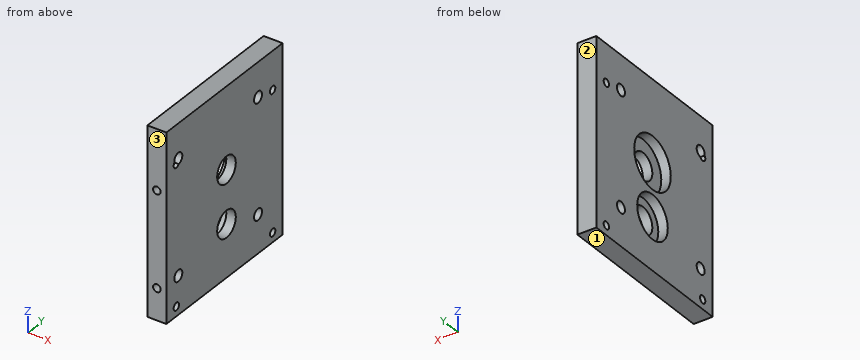
```python
from build123d import *

# Parameters (mm, degrees)
SKETCH1_W           = 20
SKETCH1_H           = 196
BOSS_EXTRUDE1_DEPTH = 175
SKETCH2_R           = 27.5
SKETCH2_R_2         = 23
CUT_EXTRUDE1_DEPTH  = 10
SKETCH3_R           = 14
CUT_EXTRUDE2_DEPTH  = 201.820815654
SKETCH4_R           = 4
CUT_EXTRUDE3_DEPTH  = 202.566366242
SKETCH5_R           = 6
CUT_EXTRUDE4_DEPTH  = 202.566366242
SKETCH6_R           = 4
CUT_EXTRUDE6_DEPTH  = 12


with BuildPart() as part:
    # Sketch1 → Boss-Extrude1 (new body)
    with BuildSketch(Plane(origin=(114, 0, 0), x_dir=(1, 0, 0), z_dir=(0, 1, 0))):
        with Locations((-114, 0)):
            Rectangle(SKETCH1_W, SKETCH1_H)
    extrude(amount=BOSS_EXTRUDE1_DEPTH)

    # Sketch2 → Cut-Extrude1 (cut)
    with BuildSketch(Plane.ZY.offset(10)):
        with Locations((12.5, 90.5)):
            Circle(SKETCH2_R)
        with Locations((-43, 90.5)):
            Circle(SKETCH2_R_2)
    extrude(amount=-CUT_EXTRUDE1_DEPTH, mode=Mode.SUBTRACT)

    # Sketch3 → Cut-Extrude2 (cut, through all)
    with BuildSketch(Plane.ZY):
        with Locations((12.5, 90.5)):
            Circle(SKETCH3_R)
        with Locations((-43, 90.5)):
            Circle(SKETCH3_R)
    extrude(amount=-CUT_EXTRUDE2_DEPTH, mode=Mode.SUBTRACT)

    # Sketch4 → Cut-Extrude3 (cut, through all)
    with BuildSketch(Plane.ZY.offset(10)):
        with Locations((58, 15)):
            Circle(SKETCH4_R)
        with Locations((-88, 15)):
            Circle(SKETCH4_R)
        with Locations((-88, 160)):
            Circle(SKETCH4_R)
        with Locations((58, 160)):
            Circle(SKETCH4_R)
    extrude(amount=-CUT_EXTRUDE3_DEPTH, mode=Mode.SUBTRACT)

    # Sketch5 → Cut-Extrude4 (cut, through all)
    with BuildSketch(Plane.ZY.offset(10)):
        with Locations((62, 138)):
            Circle(SKETCH5_R)
        with Locations((62, 18)):
            Circle(SKETCH5_R)
        with Locations(Location((-58, 138, 0), (0, 0, 180))):
            Circle(SKETCH5_R)
        with Locations((-58, 18)):
            Circle(SKETCH5_R)
    extrude(amount=-CUT_EXTRUDE4_DEPTH, mode=Mode.SUBTRACT)

    # Sketch6 → Cut-Extrude6 (cut)
    with BuildSketch(Plane.XZ):
        with Locations(Location((0, -65, 0), (0, 0, 270))):
            Circle(SKETCH6_R)
        with Locations(Location((0, 35, 0), (0, 0, 90))):
            Circle(SKETCH6_R)
    extrude(amount=-CUT_EXTRUDE6_DEPTH, mode=Mode.SUBTRACT)


solid = part.part
```
Verification items for the finished model (mm, model axes). Face numbers are marked on the shaded views. Give positions to 0.01 mm unless a question says otherwise; leave off trailing zeros. Loops run counter-clockwise (first coordinate to the right, second up) from the corner with the lowest first, then second, coordinate; pieces in that order, holes last.
1. Section check B-B, the plane y = 15. Enter the section's corners in (x, z), then the cut area to 3 significant figures.
2. Section check D-D, the plane z = 13. Enter the section's corners in (x, y), then the cut area to 3 significant figures.
3. Thickness scan on line 1 (Z direction, x = -5, y = 138.5); line 2 (Y direction, x = -3, z = -43); line 3 (Z direction, x = 9, y = 159). Record the ranges inside material, lowest first.
4. Section check C-C, the plane x = 6.25. Count the separate pieces of the cut face and the enclosed holes in it, then the cut area to 3 significant figures.
5. Mould release check, pull along Y, two halves, no side actions. Record for the marked faces 1, 2 and 3: released by +Y, released by -Y, zero draft, split by the parting line, or undercut.
6. Go/stop test with a flat-tipped pin: pin 1 Ø2.5 at (x, z) = (-2, -64.5) entering from -Y. Record where the tip stops, or that it passes through.
7. Section check A-A, the plane y = 138. Enter the section's corners in (x, z).
Geometry says:
1. outline: (-10, -98) - (10, -98) - (10, -92) - (-10, -92) - close; (-10, -84) - (10, -84) - (10, -63.2) - (-10, -63.2) - close; (-10, -52.8) - (10, -52.8) - (10, 54) - (-10, 54) - close; (-10, 67.2) - (10, 67.2) - (10, 98) - (-10, 98) - close
1. area: 3,290 mm2
2. outline: (-10, 0) - (10, 0) - (10, 76.51) - (0, 76.51) - (0, 63) - (-10, 63) - close; (-10, 118) - (0, 118) - (0, 104.49) - (10, 104.49) - (10, 175) - (-10, 175) - close
2. area: 2,670 mm2
3. line 1: z = -98 to -63.98, -52.02 to 56.02, 67.98 to 98
3. line 2: y = 0 to 67.5, 113.5 to 175
3. line 3: z = -98 to -91.87, -84.13 to 54.13, 61.87 to 98
4. separate pieces: 1
4. enclosed holes: 9
4. area: 32,400 mm2
5. face 1: zero draft
5. face 2: released by +Y
5. face 3: released by -Y
6. pin 1: stops at y = 12
7. outline: (-10, -98) - (10, -98) - (10, -64) - (-10, -64) - close; (-10, -52) - (10, -52) - (10, 56) - (-10, 56) - close; (-10, 68) - (10, 68) - (10, 98) - (-10, 98) - close
